The model under review builds one solid part; all positions refer to its coordinate system, in mm. Round coordinates to 2 decimals unless told otherwise and drop trailing zeros. Loops run counter-clockwise (first coordinate to the right, second up) from the corner with the lowest first, then second, coordinate; pieces in that order, holes last. Notation, with made-up numbers: M 48.25,88.5 L 86.25,88.5 A30 ccw 86.25,110.5 Z; hole C 22,87 d9. An arc over 180 degrees is marked long. Answer in a Markdown table with one row per item. Add a question column.
Autodesk Inventor part; units mm, degrees
ref_plane "YZ Plane" through (0, 0, 0) normal (1, 0, 0) x (0, 1, 0)
ref_plane "XZ Plane" through (0, 0, 0) normal (0, 1, 0) x (-1, 0, 0)
ref_plane "XY Plane" through (0, 0, 0) normal (0, 0, 1) x (1, 0, 0)
sketch "Boceto1" plane through (0, 0, 0) normal (0, 0, 1) x (1, 0, 0)
  line L0 (200, -155) -> (-200, -155)
  line L1 (-200, -155) -> (-200, 105)
  line L2 (-200, 105) -> (-105, 105)
  line L3 (-105, 105) -> (-105, 200)
  line L4 (-105, 200) -> (-10, 200)
  line L5 (-10, 200) -> (-10, 105)
  line L6 (200, -155) -> (200, -5)
  line L7 (200, -5) -> (-10, 105)
  line L8 (-27.6071, -98.5) -> (29.3929, -98.5)
  line L9 (29.3929, -98.5) -> (29.3929, -41.5)
  line L10 (29.3929, -41.5) -> (-27.6071, -41.5)
  line L11 (-27.6071, -41.5) -> (-27.6071, -98.5)
  line L12 (-27.6071, -98.5) -> (29.3929, -41.5) construction
  line L13 (29.3929, -98.5) -> (-27.6071, -41.5) construction
  line L14 (-20, 115) -> (-95, 115)
  line L15 (-95, 115) -> (-95, 190)
  line L16 (-95, 190) -> (-20, 190)
  line L17 (-20, 190) -> (-20, 115)
  line L18 (-20, 115) -> (-95, 190) construction
  line L19 (-95, 115) -> (-20, 190) construction
  point P0 (0.8929, -70)
  point P1 (-57.5, 152.5)
  dimension "d2" = 260
  dimension "d3" = 95
  dimension "d4" = 95
  dimension "d5" = 150
  dimension "d6" = 400
  dimension "d7" = 57
  dimension "d8" = 57
  dimension "d10" = 75
  dimension "d11" = 75
extrude "Extrusión1" add sketch "Boceto1" along normal blind 6
fillet "Empalme1" radius 6 16 edges at (-10, 105, 3) (-10, 200, 3) (200, -5, 3) (200, -155, 3) (-200, -155, 3) (-200, 105, 3) (-105, 105, 3) (-105, 200, 3) (-95, 190, 3) (-20, 190, 3) (-20, 115, 3) (-95, 115, 3) (-27.6071, -41.5, 3) (29.3929, -41.5, 3) (29.3929, -98.5, 3) (-27.6071, -98.5, 3)
sketch "Boceto2" plane through (0, 0, 6) normal (0, 0, 1) x (1, 0, 0)
  line L0 (10, -110) -> (-10, -110)
  line L1 (-10, -110) -> (-10, -104)
  line L2 (-10, -104) -> (10, -104)
  line L3 (10, -104) -> (10, -110)
  line L4 (10, -110) -> (-10, -104) construction
  line L5 (-10, -110) -> (10, -104) construction
  line L6 (-194, -155) -> (194, -155)
  line L7 (-50, -110) -> (-70, -110)
  line L8 (-70, -110) -> (-70, -104)
  line L9 (-70, -104) -> (-50, -104)
  line L10 (-50, -104) -> (-50, -110)
  line L11 (-50, -110) -> (-70, -104) construction
  line L12 (-70, -110) -> (-50, -104) construction
  line L13 (70, -110) -> (50, -110)
  line L14 (50, -110) -> (50, -104)
  line L15 (50, -104) -> (70, -104)
  line L16 (70, -104) -> (70, -110)
  line L17 (70, -110) -> (50, -104) construction
  line L18 (50, -110) -> (70, -104) construction
  circle A0 centre (-170, -107) radius 4
  line L19 (-190, -110) -> (-210, -110)
  line L20 (-210, -110) -> (-210, -104)
  line L21 (-210, -104) -> (-190, -104)
  line L22 (-190, -104) -> (-190, -110)
  line L23 (-200, -149) -> (-200, 99)
  line L24 (-190, -110) -> (-210, -104) construction
  line L25 (-210, -110) -> (-190, -104) construction
  circle A1 centre (-80, -95) radius 3
  circle A2 centre (-80, -51) radius 3
  circle A3 centre (-170, -80) radius 3
  circle A4 centre (-170, -60) radius 3
  line L26 (0, 0) -> (0, -107)
  circle A5 centre (170, -107) radius 4
  line L27 (190, -110) -> (210, -110)
  line L28 (210, -110) -> (210, -104)
  line L29 (210, -104) -> (190, -104)
  line L30 (190, -104) -> (190, -110)
  circle A6 centre (80, -95) radius 3
  circle A7 centre (80, -51) radius 3
  line L31 (194, -155) -> (-194, -155)
  arc A8 (29.2, -155) -> (-29.2, -155) centre (0, -182.3379) ccw
  line L32 (-29.2, -155) -> (29.2, -155)
  point P0 (-60, -107)
  point P1 (60, -107)
  point P2 (-200, -107)
  dimension "d15" = 20
  dimension "d16" = 6
  dimension "d17" = 48
  dimension "d18" = 20
  dimension "d19" = 60
  dimension "d20" = 20
  dimension "d21" = 60
  dimension "d22" = 8
  dimension "d23" = 20
  dimension "d24" = 6
  dimension "d25" = 110
  dimension "d26" = 6
  dimension "d27" = 20
  dimension "d28" = 12
  dimension "d29" = 6
  dimension "d30" = 44
  dimension "d31" = 6
  dimension "d32" = 6
  dimension "d33" = 40
  dimension "d36" = 6
  dimension "d37" = 6
extrude "Extrusión2" cut sketch "Boceto2" against normal through all
properties part number "EXTERNAL SIDE PLATE" material "Acero, carbono"
1. Take a section at B-B, the plane y = 20. State the section outline as (x, z) points, and give its area (3 significant figures).
2. Take a section at C-C, the plane x = 155. State the section outline as (y, z) points, and give its area (3 significant figures).
3. Mouldability with a two-part tool opening along X and no side actions: class faces 1 (the flat face through (-3, -14, 0)), 2 (the flat face through (96.425, 49.254, 2.958)), 3 (the cylindrical face through (0.46, -142.34, 3.04)) as released by +X, released by -X, zero draft, split by the parting line, or undercut.
4. For pin 1 Ø1 at (y, z) = (131.5, 3) entering from -X; pin 2 Ø3 at (y, z) = (152.5, 2.5) entering from +X; pin 3 Ø1.5 at (y, z) = (50, 3) entering from +X, all flat-tipped, find the tip position at first contact; note any pin that passes through.
5. Take a section at A-A, the plane z = 2.55. State how many separate pieces and enclosed holes the cut face has, and give its area (3 significant figures).
6. To check wall thickness, follow probe 1 along Y at (x, z) = (-170, 3.5); probe 2 along Y at (x, z) = (-31, 1.8); probe 3 along X at (y, z) = (148, 4.4). State the ranges of each line that lie inside material, in increasing order.
Check sheet entries:
| question | item | result |
|---|---|---|
| 1 | outline | M -200,0 L 152.27,0 L 152.27,6 L -200,6 Z |
| 1 | area | 2,110 mm^2 |
| 2 | outline | M -155,0 L 18.57,0 L 18.57,6 L -155,6 Z |
| 2 | area | 1,040 mm^2 |
| 3 | face 1 | zero draft |
| 3 | face 2 | released by +X |
| 3 | face 3 | undercut |
| 4 | pin 1 | stops at x = -105 |
| 4 | pin 2 | stops at x = -10 |
| 4 | pin 3 | stops at x = 96.43 |
| 5 | separate pieces | 1 |
| 5 | enclosed holes | 13 |
| 5 | area | 91,400 mm^2 |
| 6 | probe 1 | y = -155 to -111, -103 to -83, -77 to -63, -57 to 105 |
| 6 | probe 2 | y = -155 to 115, 190 to 200 |
| 6 | probe 3 | x = -105 to -95, -20 to -10 |
